Geometry check sheet. Reference: drawing and pictorial views, mm from the part's lowest x, y, z. A direction names the side the tool comes from. Round coordinates to 2 decimals unless told otherwise and drop trailing zeros. Loops run counter-clockwise (first coordinate to the right, second up) from the corner with the lowest first, then second, coordinate; pieces in that order, holes last. Notation, with made-up numbers: (10.5, 46) - (26.5, 46) arc R10 cw to (26.5, 54) - close; hole circle Ø10 at (-12.5, 54). An arc over 180 degrees is marked (long way). Answer as CSV lines item,"result". Start each with the question number.
1) Cross-section at B-B on x = 42. Record the boundary of the cut face in (y, z), and give its area (3 significant figures).
2) Cross-section at A-A on z = 15.92. State how many separate pieces and enclosed holes the cut face has.
3) Depth check by flat-ended pin: P1, Ø3.5, axis at x = 42, z = 8, coming from the -Y side; P2, Ø8.5, axis at x = 51, z = 20.5, coming from the +Y side; P3, Ø8, axis at x = 25.5, z = 17, coming from the -Y side; P4, Ø12, axis at x = 7, y = 25.5, coming from the +Z side. Enter the tip coordinate at first touch or a pass-through.
4) Access from +Z, -Z, +X, -X, +Y, -Y to the whole of each face (thin tool, end or side, straight path). Record for the marked faces 1, 2, 3, 4 and 5.
5) Cross-section at D-D on z = 8. Record the boundary of the cut face in (x, y), and give its area (3 significant figures).
6) Thickness scan on line 1 along Z through (x, y) = (52, 8); line 2 along X through (y, z) = (13, 16) (1 decimal); line 3 along Z through (x, y) = (4.5, 3) (1 decimal). Record the ranges inside material, lowest first.
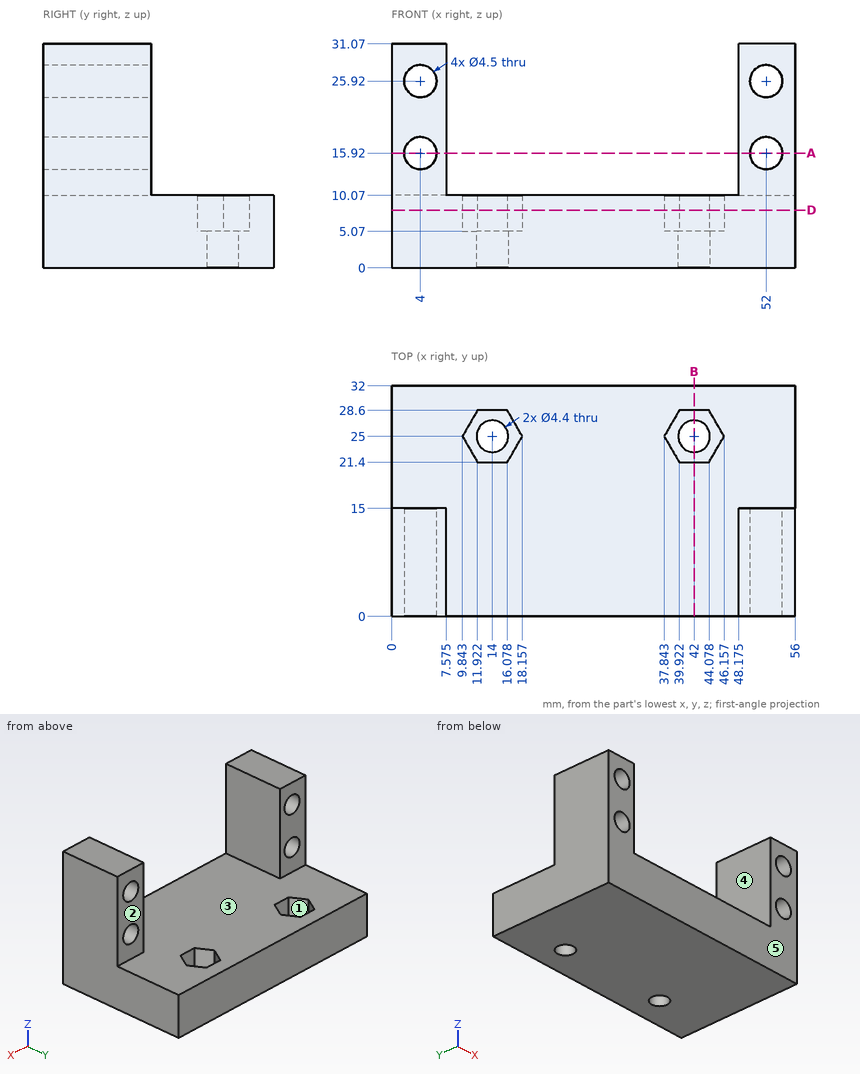
Answer block:
1,outline,"(0, 0) - (22.8, 0) - (22.8, 5.07) - (21.4, 5.07) - (21.4, 10.07) - (0, 10.07) - close; (27.2, 0) - (32, 0) - (32, 10.07) - (28.6, 10.07) - (28.6, 5.07) - (27.2, 5.07) - close"
1,area,"264 mm^2"
2,separate pieces,"4"
2,enclosed holes,"0"
3,P1,"stops at y = 0"
3,P2,"stops at y = 15"
3,P3,"passes through"
3,P4,"stops at z = 10.07"
4,face 1,"+Z"
4,face 2,"+Z, +X, -X, +Y"
4,face 3,"+Z, +Y"
4,face 4,"+Z, +Y, -Y"
4,face 5,"+Z, -Z, +X, -X, -Y"
5,outline,"(0, 0) - (56, 0) - (56, 32) - (0, 32) - close; hole (9.84, 25) - (11.92, 21.4) - (16.08, 21.4) - (18.16, 25) - (16.08, 28.6) - (11.92, 28.6) - close; hole (37.84, 25) - (39.92, 21.4) - (44.08, 21.4) - (46.16, 25) - (44.08, 28.6) - (39.92, 28.6) - close"
5,area,"1,700 mm^2"
6,line 1,"z = 0 to 13.67, 18.17 to 23.67, 28.17 to 31.07"
6,line 2,"x = 0 to 1.8, 6.2 to 7.6, 48.2 to 49.8, 54.2 to 56"
6,line 3,"z = 0 to 13.7, 18.1 to 23.7, 28.1 to 31.1"
